Read the model definition and answer for the solid it produces. Units are mm, in the model's axes. Give positions to 0.01 mm unless a question says otherwise; leave off trailing zeros. Write each loop counter-clockwise with the first axis right and the second up, starting at its lowest first coordinate (ties: lowest second). Pieces come first, ordered by that corner, then holes. Notation, with made-up numbers: (8.5, 88.25) - (23.5, 88.25) arc R19 cw to (23.5, 93.25) - close; hole circle Ø2 at (-25.5, -4.5). An arc over 180 degrees is marked (long way). Use CSV: the item, a comma, the result in double quotes. Start each with the question number.
from build123d import *

# Parameters (mm, degrees)
F0_W     = 400.05
F0_H     = 762
F1_DEPTH = 25.4
F2_W     = 390.525
F2_H     = 762
F3_DEPTH = 25.4


with BuildPart() as f1:
    # F0 (on Right) → F1 (new body)
    with BuildSketch(Plane.YZ):
        Rectangle(F0_W, F0_H)
    extrude(amount=F1_DEPTH)

    # F2 (on Front) → F3 (join)
    with BuildSketch(Plane.XZ):
        with Locations((195.2625, -0.671017)):
            Rectangle(F2_W, F2_H)
    extrude(amount=F3_DEPTH)


solid = f1.part
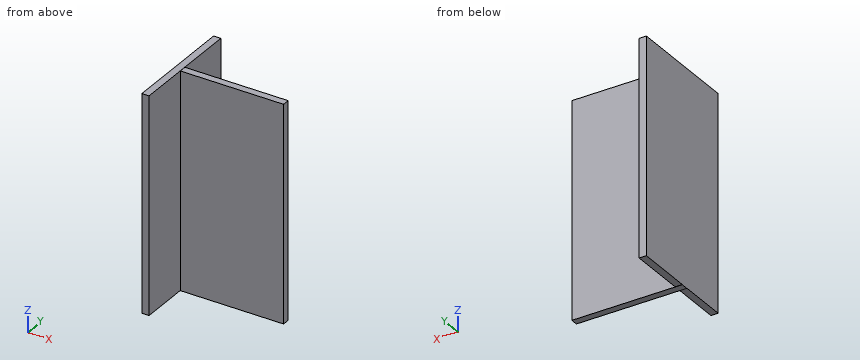
(1) Consider probe 1 along Y at (x, z) = (81, 316.5); probe 2 along Z at (x, y) = (318.5, -14); probe 3 along X at (y, z) = (175, 283). Determine where each line is inside the solid, lowest interval first.
(2) Given P1, Ø6, axis at x = 170, y = -28.5, coming from the -Z side; P2, Ø2, axis at y = -102.5, z = 198.5, coming from the +X side; P3, Ø1, axis at x = 282.5, z = -293, coming from the +Y side; P4, Ø12.5, axis at x = 249, y = -9, coming from the +Z side, each flat-ended and moving along its own axis, determine where each tip first touches the part or whether it passes through.
(3) The part is cut by section B-B on x = 330. Write down the section's boundary in (y, z).
(4) The part is cut by section A-A on z = 206. Write down the section's boundary in (x, y) (3 decimals), plus the area to 3 significant figures.
(5) The part is cut by section C-C on y = -60. Write down the section's boundary in (x, z), plus the area to 3 significant figures.
Reported:
1,probe 1,"-25.4 to 0"
1,probe 2,"-381.67 to 380.33"
1,probe 3,"0 to 25.4"
2,P1,"through"
2,P2,"x = 25.4"
2,P3,"y = 0"
2,P4,"z = 380.33"
3,outline,"(-25.4, -381.67) - (0, -381.67) - (0, 380.33) - (-25.4, 380.33) - close"
4,outline,"(0, -200.025) - (25.4, -200.025) - (25.4, -25.4) - (390.525, -25.4) - (390.525, 0) - (25.4, 0) - (25.4, 200.025) - (0, 200.025) - close"
4,area,"19,400 mm²"
5,outline,"(0, -381) - (25.4, -381) - (25.4, 381) - (0, 381) - close"
5,area,"19,400 mm²"
